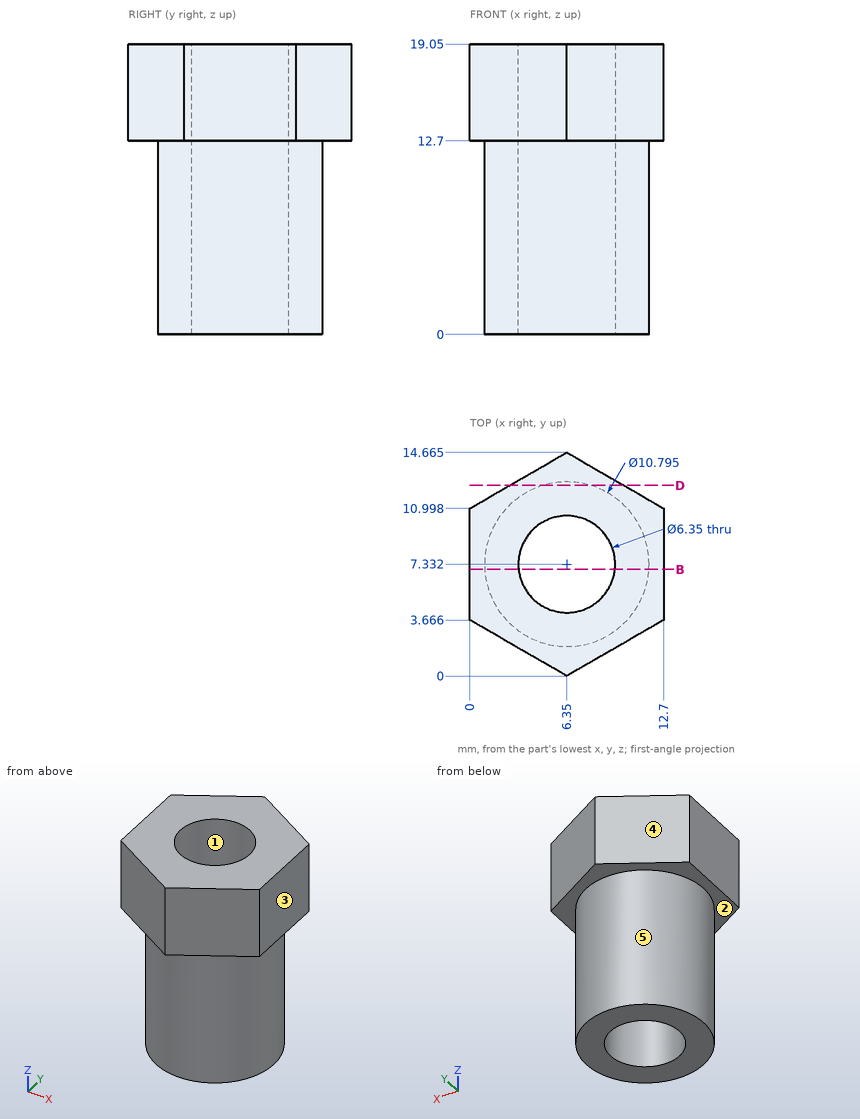
Geometry check sheet. Reference: drawing and pictorial views, mm from the part's lowest x, y, z. A direction names the side the tool comes from. Round coordinates to 2 decimals unless told otherwise and drop trailing zeros. Loops run counter-clockwise (first coordinate to the right, second up) from the corner with the lowest first, then second, coordinate; pieces in that order, holes last. Notation, with made-up numbers: (22.5, 19.5) -> (50.5, 19.5) arc R8 cw to (50.5, 27.5) -> close; hole circle Ø6 at (-3.75, 86). An arc over 180 degrees is marked (long way). Use a Markdown table: item, result.
(1) Sectioned sample at B-B (y = 7). Enter the section's corners in (x, z).
Calculated:
| item | result |
|---|---|
| outline | (0, 12.7) -> (0.96, 12.7) -> (0.96, 0) -> (3.19, 0) -> (3.19, 19.05) -> (0, 19.05) -> close; (9.51, 0) -> (11.74, 0) -> (11.74, 12.7) -> (12.7, 12.7) -> (12.7, 19.05) -> (9.51, 19.05) -> close |
(2) Scan lines: probe 1 along Y at (x, z) = (6.5, 9); probe 2 along X at (y, z) = (7.5, 17); probe 3 along Y at (x, z) = (7, 11.25) (1 decimal). Record each from-to range of solid material in increasing order.
Calculated:
| item | result |
|---|---|
| probe 1 | 1.94 to 4.16, 10.5 to 12.73 |
| probe 2 | 0 to 3.18, 9.52 to 12.7 |
| probe 3 | 2 to 4.2, 10.4 to 12.7 |
(3) Mould release check, pull along X, two halves, no side actions. Record for the marked faces 1, 2 and 3: released by +X, released by -X, zero draft, split by the parting line, or undercut.
Calculated:
| item | result |
|---|---|
| face 1 | undercut |
| face 2 | zero draft |
| face 3 | released by +X |
(4) Set-up check for the marked faces 4 and 5: record each of +Z, -Z, +X, -X, +Y, -Y from which the full face is reachable in a straight line by a thin tool's end or side.
Calculated:
| item | result |
|---|---|
| face 4 | +Z, -Z, -X, +Y |
| face 5 | -Z |
(5) Sectioned sample at D-D (y = 12.5). Enter the section's corners in (x, z).
Calculated:
| item | result |
|---|---|
| outline | (2.6, 12.7) -> (4.79, 12.7) -> (4.79, 0) -> (7.91, 0) -> (7.91, 12.7) -> (10.1, 12.7) -> (10.1, 19.05) -> (2.6, 19.05) -> close |
(6) Go/stop test with flat-tipped pins: P1, Ø3, axis at x = 4, z = 8.5, coming from the -Y side; P2, Ø5, axis at x = 8.5, z = 3, coming from the -Y side (1 decimal); P3, Ø2, axis at y = 8, z = 11.5, coming from the +X side. Record where each tip stops, or that it passes through.
Calculated:
| item | result |
|---|---|
| P1 | y = 2 |
| P2 | y = 1.9 |
| P3 | x = 11.75 |
